from build123d import *

# Parameters (mm, degrees)
SKETCH1_W             = 5
SKETCH1_H             = 40
SKETCH1_R             = 1.3
BOSS_EXTRUDE1_DEPTH   = 11
BOSS_EXTRUDE1_2_DEPTH = 11
SKETCH2_W             = 39.3
SKETCH2_H             = 6
BOSS_EXTRUDE2_DEPTH   = 25
BOSS_EXTRUDE3_DEPTH   = 4.8
FILLET1_R             = 1
SKETCH4_R             = 3
CUT_EXTRUDE1_DEPTH    = 34
FILLET2_R             = 10
FILLET3_R             = 8


with BuildPart() as part:
    # Sketch1 → Boss-Extrude1 (new body)
    with BuildSketch(Plane(origin=(0, 0, 0), x_dir=(0, 0, -1), z_dir=(1, 0, 0))):
        with Locations((-17.15, 20)):
            Rectangle(SKETCH1_W, SKETCH1_H)
        with Locations((-17.3, 32.5)):
            Circle(SKETCH1_R, mode=Mode.SUBTRACT)
        with Locations((-17.3, 10.5)):
            Circle(SKETCH1_R, mode=Mode.SUBTRACT)
    extrude(amount=BOSS_EXTRUDE1_DEPTH)



with BuildPart() as body_2:
    # Sketch1 → Boss-Extrude1 2 (new body)
    with BuildSketch(Plane(origin=(0, 0, 0), x_dir=(0, 0, -1), z_dir=(1, 0, 0))):
        with Locations((17.15, 20)):
            Rectangle(SKETCH1_W, SKETCH1_H)
        with Locations((17.3, 10.5)):
            Circle(SKETCH1_R, mode=Mode.SUBTRACT)
        with Locations((17.3, 32.5)):
            Circle(SKETCH1_R, mode=Mode.SUBTRACT)
    extrude(amount=BOSS_EXTRUDE1_2_DEPTH)


with BuildPart() as part_1:
    add(part.part)

    add(body_2.part)  # Boss-Extrude2 merges body 2
    # Sketch2 → Boss-Extrude2 (add)
    with BuildSketch(Plane(origin=(11, 0, 0), x_dir=(0, 0, -1), z_dir=(1, 0, 0))):
        with Locations((0, 3)):
            Rectangle(SKETCH2_W, SKETCH2_H)
    extrude(amount=BOSS_EXTRUDE2_DEPTH)

    # Sketch3 → Boss-Extrude3 (add)
    with BuildSketch(Plane(origin=(11, 0, 0), x_dir=(0, 0, -1), z_dir=(1, 0, 0))):
        Polygon((-14.65, 22.5), (-12.65, 22.5), (-12.65, 0), (-5.65, 0), (-5.65, 22.5), (5.65, 22.5), (5.65, 0), (12.65, 0), (12.65, 22.5), (14.65, 22.5), (14.65, 28.5), (-14.65, 28.5), align=None)
    extrude(amount=-BOSS_EXTRUDE3_DEPTH)

    # Fillet1
    fillet1_edges = [part_1.edges().sort_by_distance(p)[0] for p in [
        (11, 6, 17.15),
        (11, 6, -17.15),
    ]]
    fillet(fillet1_edges, radius=FILLET1_R)

    # Sketch4 → Cut-Extrude1 (cut)
    with BuildSketch(Plane(origin=(0, 6, 0), x_dir=(1, 0, 0), z_dir=(0, 1, 0))):
        with Locations((28, 12.5)):
            Circle(SKETCH4_R)
        with Locations((28, -12.5)):
            Circle(SKETCH4_R)
    extrude(amount=-CUT_EXTRUDE1_DEPTH, mode=Mode.SUBTRACT)

    # Fillet2
    fillet2_edges = [part_1.edges().sort_by_distance(p)[0] for p in [
        (11, 6, 9.15),
        (11, 6, -9.15),
    ]]
    fillet(fillet2_edges, radius=FILLET2_R)

    # Fillet3
    fillet3_edges = [part_1.edges().sort_by_distance(p)[0] for p in [
        (8.6, 28.5, 14.65),
        (8.6, 28.5, -14.65),
    ]]
    fillet(fillet3_edges, radius=FILLET3_R)


solid = part_1.part
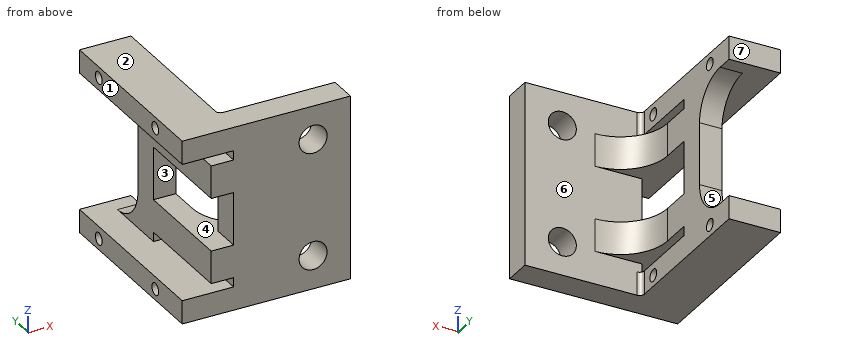
Here's how the part is built. I have some questions about the finished solid (model axes, mm). Face numbers are marked on the shaded views. A direction names the side the tool comes from. Give positions to 0.01 mm unless a question says otherwise; leave off trailing zeros. Write each loop counter-clockwise with the first axis right and the second up, starting at its lowest first coordinate (ties: lowest second). Pieces come first, ordered by that corner, then holes. Notation, with made-up numbers: (32, 54) -> (52, 54) arc R16 ccw to (52, 79) -> close; hole circle Ø7 at (43, 21.25). An arc over 180 degrees is marked (long way). Use one line per item in the form item = value. Start each with the question number.
1. On a 3-axis mill with a long thin cutter (end or side, diameter ignored), from which of +Z, -Z, +X, -X, +Y, -Y can I reach the whole of each face in a straight line? I mean the marked faces 4, 5, 6 and 7. Say none if no direction works.
2. Imagine slicing it at A-A on x = 5. List the corners of the cut face in (y, z) for me, plus the area to 3 significant figures.
3. Imagine slicing it at D-D on y = 32.5. List the corners of the cut face in (x, z) for me, plus the area to 3 significant figures.
4. Will these pins go through, and if not, where does the flat tip stop? pin 1 Ø1 at (x, z) = (9, 13.5) entering from -Y; pin 2 Ø6 at (y, z) = (15, 10) entering from +X; pin 3 Ø3 at (x, z) = (21, -11) entering from +Y.
5. If I drill on L1, parallel to Y at x = 7, z = -17.3; L2, parallel to Z at x = 28, y = 2.9; L3, parallel to Z at x = 4, y = 10, over which ranges is the centre line in solid material (lowest first)?
6. Thinking about a two-plate mould opening in Z: for the marked faces 1, 2 and 3, which applies, +Z half, -Z half, draft (parallel to the pull), parting line (faces both ways), or undercut?
7. Imagine slicing it at B-B on z = 17.3. List the corners of the cut face in (x, y) for me.
8. Imagine slicing it at C-C on x = 28. List the corners of the cut face in (y, z) for me, plus the area to 3 significant figures.
Entries:
q1.face_4 = -X
q1.face_5 = +X, -X, +Y
q1.face_6 = +X, +Y
q1.face_7 = +Z, -Z, +X, -X, +Y
q2.outline = (0, -19.65) -> (40, -19.65) -> (40, -14.65) -> (0, -14.65) -> close; (0, 14.65) -> (40, 14.65) -> (40, 19.65) -> (0, 19.65) -> close; hole circle Ø2.6 at (10.5, -17.3); hole circle Ø2.6 at (10.5, 17.3); hole circle Ø2.6 at (32.5, -17.3); hole circle Ø2.6 at (32.5, 17.3)
q2.area = 379 mm²
q3.outline = (0, -19.65) -> (11, -19.65) -> (11, -18.6) -> (0, -18.6) -> close; (0, -16) -> (11, -16) -> (11, -13.58) -> (6.2, -13.58) -> (6.2, -14.65) -> (0, -14.65) -> close; (0, 14.65) -> (6.2, 14.65) -> (6.2, 13.58) -> (11, 13.58) -> (11, 16) -> (0, 16) -> close; (0, 18.6) -> (11, 18.6) -> (11, 19.65) -> (0, 19.65) -> close
q3.area = 63.1 mm²
q4.pin_1 = 22.5
q4.pin_2 = 11.83
q4.pin_3 = 6.11
q5.L1 = 0 to 9.2, 11.8 to 31.2, 33.8 to 40
q5.L2 = -19.65 to -15.5, -9.5 to 9.5, 15.5 to 19.65
q5.L3 = -19.65 to -18.5, -16.1 to -14.65, 14.65 to 16.1, 18.5 to 19.65
q6.face_1 = draft
q6.face_2 = +Z half
q6.face_3 = undercut
q7.outline = (0, 0) -> (36, 0) -> (36, 6) -> (12, 6) arc R1 cw to (11, 7) -> (11, 9.2) -> (0, 9.2) -> close; (0, 11.8) -> (11, 11.8) -> (11, 31.2) -> (0, 31.2) -> close; (0, 33.8) -> (11, 33.8) -> (11, 40) -> (0, 40) -> close
q8.outline = (0, -19.65) -> (6, -19.65) -> (6, -15.5) -> (0, -15.5) -> close; (0, -9.5) -> (6, -9.5) -> (6, 9.5) -> (0, 9.5) -> close; (0, 15.5) -> (6, 15.5) -> (6, 19.65) -> (0, 19.65) -> close
q8.area = 164 mm²
